Input: dimensioned drawing with shaded views. Units: mm. Origin: part minimum x, y, z. Coordinates: 2 decimals unless noted, no trailing zeros. Loops run counter-clockwise (first coordinate to the right, second up) from the corner with the lowest first, then second, coordinate; pieces in that order, holes last.
(1) Section C-C, the plane z = 75.5. Return loops of the section in (x, y), then the cut area to 3 significant figures.
(2) Section B-B, the plane z = 224.5. Return loops of the section in (x, y), then the cut area to 3 significant figures.
(3) Section A-A, the plane x = 225. Return loops of the section in (y, z), then the cut area to 3 significant figures.
(4) Line query: L1, parallel to X at y = 2.85, z = 75.5; L2, parallel to X at y = 1.5, z = 224.5; L3, parallel to Z at x = 343.5, y = 0.85. Output: solid intervals per line, ascending.
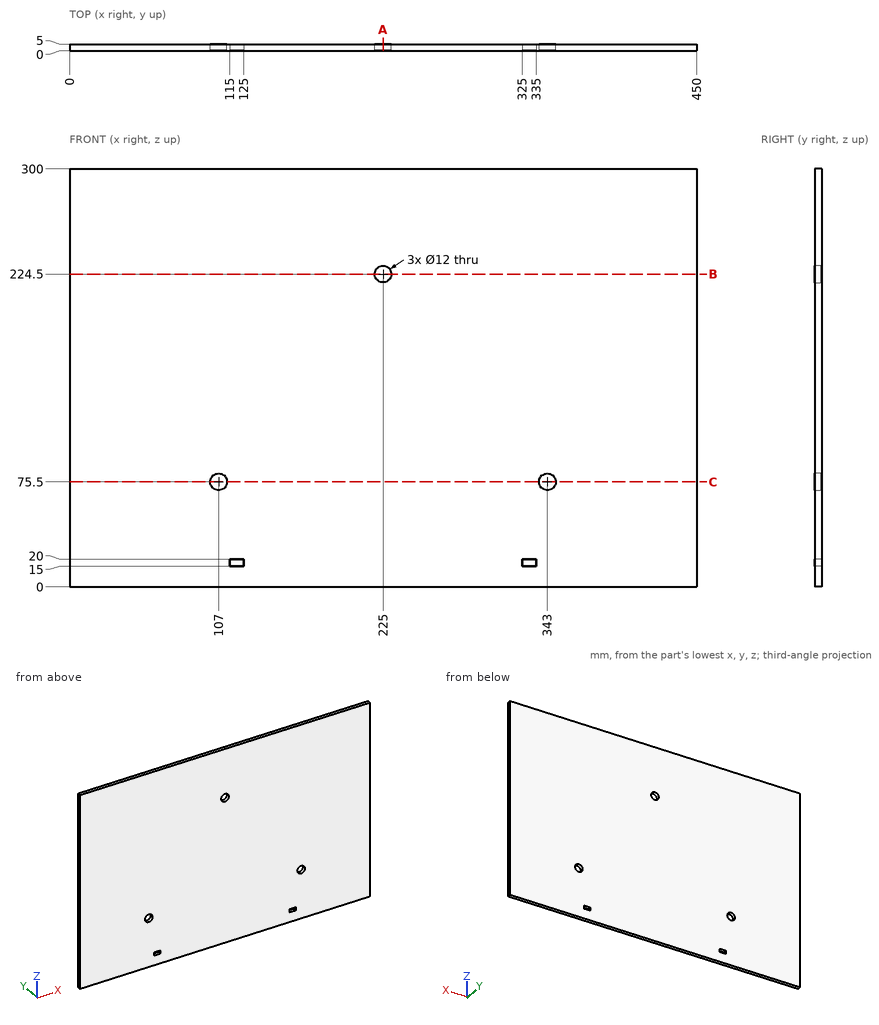
Report:
1. outline: (0, 0) - (101, 0) - (101, 5) - (0, 5) - close; (113, 0) - (337, 0) - (337, 5) - (113, 5) - close; (349, 0) - (450, 0) - (450, 5) - (349, 5) - close
1. area: 2,130 mm2
2. outline: (0, 0) - (219, 0) - (219, 5) - (0, 5) - close; (231, 0) - (450, 0) - (450, 5) - (231, 5) - close
2. area: 2,190 mm2
3. outline: (0, 0) - (5, 0) - (5, 218.5) - (0, 218.5) - close; (0, 230.5) - (5, 230.5) - (5, 300) - (0, 300) - close
3. area: 1,440 mm2
4. L1: x = 0 to 101, 113 to 337, 349 to 450
4. L2: x = 0 to 219, 231 to 450
4. L3: z = 0 to 69.52, 81.48 to 300
